```python
from build123d import *

# Parameters (mm, degrees)
SKETCH1_W           = 6
SKETCH1_H           = 5
BOSS_EXTRUDE1_DEPTH = 5
CUT_EXTRUDE1_DEPTH  = 2
CUT_EXTRUDE2_DEPTH  = 2
SKETCH5_W           = 1
SKETCH5_H           = 2
CUT_EXTRUDE3_DEPTH  = 5
CUT_EXTRUDE4_DEPTH  = 2
CUT_EXTRUDE5_DEPTH  = 2
CUT_EXTRUDE6_DEPTH  = 1


with BuildPart() as part:
    # Sketch1 → Boss-Extrude1 (new body)
    with BuildSketch(Plane.XY):
        with Locations((3, 2.5)):
            Rectangle(SKETCH1_W, SKETCH1_H)
    extrude(amount=BOSS_EXTRUDE1_DEPTH)

    # Sketch2 → Cut-Extrude1 (cut)
    with BuildSketch(Plane(origin=(6, 0, 0), x_dir=(0, 0, -1), z_dir=(1, 0, 0))):
        Polygon((0, 2), (-1, 2), (-5, 0), (0, 0), align=None)
    extrude(amount=-CUT_EXTRUDE1_DEPTH, mode=Mode.SUBTRACT)

    # Sketch4 → Cut-Extrude2 (cut)
    with BuildSketch(Plane.ZY):
        Polygon((1, 0), (5, 2), (5, 0), align=None)
    extrude(amount=-CUT_EXTRUDE2_DEPTH, mode=Mode.SUBTRACT)

    # Sketch5 → Cut-Extrude3 (cut)
    with BuildSketch(Plane(origin=(0, 5, 0), x_dir=(1, 0, 0), z_dir=(0, 1, 0))):
        with Locations((0.5, -4)):
            Rectangle(SKETCH5_W, SKETCH5_H)
    extrude(amount=-CUT_EXTRUDE3_DEPTH, mode=Mode.SUBTRACT)

    # Sketch6 → Cut-Extrude4 (cut)
    with BuildSketch(Plane.XY.offset(5)):
        Polygon((4, 5), (6, 3), (6, 5), align=None)
    extrude(amount=-CUT_EXTRUDE4_DEPTH, mode=Mode.SUBTRACT)

    # Sketch7 → Cut-Extrude5 (cut)
    with BuildSketch(Plane.XY.offset(5)):
        Polygon((4, 5), (2, 3), (1, 3), (1, 5), align=None)
    extrude(amount=-CUT_EXTRUDE5_DEPTH, mode=Mode.SUBTRACT)

    # Sketch8 → Cut-Extrude6 (cut)
    with BuildSketch(Plane.XY.offset(5)):
        Polygon((3, 4), (5, 4), (4, 5), align=None)
    extrude(amount=-CUT_EXTRUDE6_DEPTH, mode=Mode.SUBTRACT)


solid = part.part
```
Can you work these out from the model? Positions are in its coordinate system, mm. A direction names the side the tool comes from. Give positions to 0.01 mm unless a question says otherwise; leave off trailing zeros. Write each loop counter-clockwise with the first axis right and the second up, starting at its lowest first coordinate (ties: lowest second). Pieces come first, ordered by that corner, then holes. Notation, with made-up numbers: (70.5, 47) - (105.5, 47) arc R7 ccw to (105.5, 55) - close; hole circle Ø11 at (41, -2). An arc over 180 degrees is marked (long way). Write item = value, one per line. Start each with the question number.
1. Imagine slicing it at B-B (y = 3.7). Please give me the cut outline in (x, z).
2. For pin 1 (0.5 mm diameter, centred on x = 5, z = 0.5, fed in from -Y); pin 2 (1 mm diameter, centred on y = 1, z = 4, fed in from -X); pin 3 (1.6 mm diameter, centred on y = 0.5, z = 2, fed in from +X), each with a flat end and sliding along its axis, tell me the tip position at first contact or that it passes through.
3. Imagine slicing it at C-C (x = 4.65). Please give me the cut outline in (y, z).
4. On a 3-axis mill with a long thin cutter (end or side, diameter ignored), from which of +Z, -Z, +X, -X, +Y, -Y can I reach the whole of each face in a straight line? I mean faces 1 (the face through (5.4, 4.5, 3)), 2 (the face through (1.208, 0.764, 2.528)), 3 (the face through (5, 1, 3)). Say none if no direction works.
5. Imagine slicing it at D-D (y = 0.5). Please give me the cut outline in (x, z).
6. Imagine slicing it at A-A (z = 4.3). Please give me the cut outline in (x, y).
7. Please list where these lines run through material, in increasing order: line 1 (Z direction, x = 0.35, y = 3.05); line 2 (Y direction, x = 5.4, z = 0.2); line 3 (Z direction, x = 3.85, y = 4.05).
Worked answers:
q1.outline = (0, 0) - (6, 0) - (6, 3) - (5.3, 3) - (5.3, 5) - (2.7, 5) - (2.7, 3) - (0, 3) - close
q2.pin_1 = 2
q2.pin_2 = 1
q2.pin_3 = 4
q3.outline = (0, 5) - (2, 1) - (2, 0) - (5, 0) - (5, 3) - (4.35, 3) - (4.35, 4) - (4, 4) - (4, 5) - close
q4.face_1 = +Z, +X, +Y
q4.face_2 = +Z, -X, -Y
q4.face_3 = -Z, +X, -Y
q5.outline = (0, 0) - (4, 0) - (4, 4) - (6, 4) - (6, 5) - (2, 5) - (2, 2) - (0, 2) - close
q6.outline = (1, 1.65) - (2, 1.65) - (2, 0) - (4, 0) - (4, 0.35) - (6, 0.35) - (6, 3) - (5, 4) - (3, 4) - (2, 3) - (1, 3) - close
q7.line_1 = 0 to 3
q7.line_2 = 2 to 5
q7.line_3 = 0 to 4
